Verification items for the finished model (mm, model axes). Face numbers are marked on the shaded views. A direction names the side the tool comes from. Coordinates: 2 decimals unless noted, no trailing zeros. Loops run counter-clockwise (first coordinate to the right, second up) from the corner with the lowest first, then second, coordinate; pieces in that order, holes last.
Q1. Access from +Z, -Z, +X, -X, +Y, -Y to the whole of each face (thin tool, end or side, straight path). Record for the marked faces 1 and 2.
Q2. Go/stop test with flat-tipped pins: P1, Ø2, axis at x = 4, y = 1, coming from the -Z side; P2, Ø2.5, axis at x = 0, z = -4.2, coming from the -Y side. Record where each tip stops, or that it passes through.
Q3. Mould release check, pull along Y, two halves, no side actions. Record for the marked faces 3, 4 and 5: +Y half, -Y half, draft (parallel to the pull), parting line (faces both ways), or undercut.
Q4. Material ranges on probe 1 along Y at (x, z) = (-3.5, -0.75); probe 2 along Z at (x, y) = (-1.25, 7); probe 3 along Z at (x, y) = (5, 4.75), recorded low to high.
Q5. Sectioned sample at B-B (x = 0). Enter the section's corners in (y, z).
Q6. Sectioned sample at A-A (y = -6). Enter the section's corners in (x, z), then the cut area to 3 significant figures.
Q7. Sectioned sample at D-D (y = 0.5). Enter the section's corners in (x, z), then the cut area to 3 significant figures.
Q8. Sectioned sample at C-C (z = -3.5). Enter the section's corners in (x, y), then the cut area to 3 significant figures.
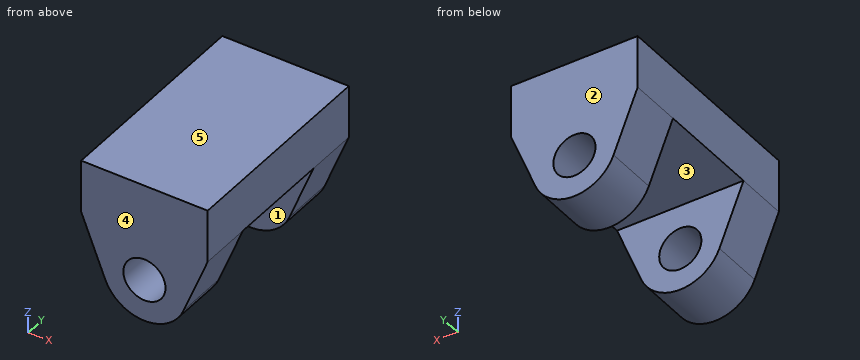
```python
from build123d import *

# Parameters (mm, degrees)
SKETCH1_W           = 12
SKETCH1_H           = 20
BOSS_EXTRUDE1_DEPTH = 5
SKETCH2_R           = 2
BOSS_EXTRUDE2_DEPTH = 5


with BuildPart() as part:
    # Sketch1 → Boss-Extrude1 (new body)
    with BuildSketch(Plane.XY):
        Rectangle(SKETCH1_W, SKETCH1_H)
    extrude(amount=BOSS_EXTRUDE1_DEPTH)

    # Sketch2 → Boss-Extrude2 (add)
    with BuildSketch(Plane(origin=(0, 10, 0), x_dir=(1, 0, 0), z_dir=(0, 1, 0))):
        with BuildLine():
            Line((-6, 0), (-3.711490956, 5.694454764))
            ThreePointArc((-3.711490956, 5.694454764), (0, 8.202866725), (3.711490956, 5.694454764))
            Line((3.711490956, 5.694454764), (6, 0))
            Line((6, 0), (-6, 0))
        make_face()
        with Locations(Location((0, 4.202866725, 0), (0, 0, 270))):
            Circle(SKETCH2_R, mode=Mode.SUBTRACT)
    boss_extrude2 = extrude(amount=-BOSS_EXTRUDE2_DEPTH)

    # Mirror1: Boss-Extrude2 across plane
    add(boss_extrude2.mirror(Plane.ZX))


solid = part.part
```
Geometry check:
1. face 1: -Z, +X, -X
1. face 2: +Z, -Z, +X, -X, +Y
2. P1: stops at z = 0
2. P2: passes through
3. face 3: undercut
3. face 4: -Y half
3. face 5: draft
4. probe 1: y = -10 to -5, 5 to 10
4. probe 2: z = -8 to -5.76, -2.64 to 5
4. probe 3: z = 0 to 5
5. outline: (-10, -8.2) - (-5, -8.2) - (-5, -6.2) - (-10, -6.2) - close; (-10, -2.2) - (-5, -2.2) - (-5, 0) - (5, 0) - (5, -2.2) - (10, -2.2) - (10, 5) - (-10, 5) - close; (5, -8.2) - (10, -8.2) - (10, -6.2) - (5, -6.2) - close
6. outline: (-6, 0) - (-3.71, -5.69) arc R4 ccw to (3.71, -5.69) - (6, 0) - (6, 5) - (-6, 5) - close; hole circle Ø4 at (0, -4.2)
6. area: 116 mm2
7. outline: (-6, 0) - (6, 0) - (6, 5) - (-6, 5) - close
7. area: 60.0 mm2
8. outline: (-4.59, -10) - (-1.87, -10) - (-1.87, -5) - (-4.59, -5) - close; (-4.59, 5) - (-1.87, 5) - (-1.87, 10) - (-4.59, 10) - close; (1.87, -10) - (4.59, -10) - (4.59, -5) - (1.87, -5) - close; (1.87, 5) - (4.59, 5) - (4.59, 10) - (1.87, 10) - close
8. area: 54.4 mm2
